```python
from build123d import *

# Parameters (mm, degrees)
F0_R     = 10.5
F1_DEPTH = 1
F2_DEPTH = 50
F3_R     = 5
F5_DEPTH = 51
F6_R     = 0.5


with BuildPart() as f1:
    # F0 (on Top) → F1 (new body)
    with BuildSketch(Plane.XY):
        with BuildLine():
            ThreePointArc((11, -3.3541019662), (10.6256868339, -1.6955824958), (10.5, 0))
            ThreePointArc((10.5, 0), (10.6256868339, 1.6955824958), (11, 3.3541019662))
            ThreePointArc((11, 3.3541019662), (-11.5, 0), (11, -3.3541019662))
        make_face()
        Circle(F0_R, mode=Mode.SUBTRACT)
        with BuildLine():
            ThreePointArc((55.5, 0), (45.6955824958, 11.3743131661), (33, 3.3541019662))
            ThreePointArc((33, 3.3541019662), (33.3743131661, 1.6955824958), (33.5, 0))
            ThreePointArc((33.5, 0), (33.3743131661, -1.6955824958), (33, -3.3541019662))
            ThreePointArc((33, -3.3541019662), (45.6955824958, -11.3743131661), (55.5, 0))
        make_face()
        with BuildLine():
            ThreePointArc((54.5, 0), (44, -10.5), (33.5, 0))
            ThreePointArc((33.5, 0), (44, 10.5), (54.5, 0))
        make_face(mode=Mode.SUBTRACT)
        Circle(F0_R)
        with BuildLine():
            ThreePointArc((32.5, 0), (22, 10.5), (11.5, 0))
            ThreePointArc((11.5, 0), (22, -10.5), (32.5, 0))
        make_face()
        with BuildLine():
            ThreePointArc((54.5, 0), (44, 10.5), (33.5, 0))
            ThreePointArc((33.5, 0), (44, -10.5), (54.5, 0))
        make_face()
        with BuildLine():
            ThreePointArc((33, 3.3541019662), (22, 11.5), (11, 3.3541019662))
            ThreePointArc((11, 3.3541019662), (11.3743131661, 1.6955824958), (11.5, 0))
            ThreePointArc((11.5, 0), (22, 10.5), (32.5, 0))
            ThreePointArc((32.5, 0), (32.6256868339, 1.6955824958), (33, 3.3541019662))
        make_face()
        with BuildLine():
            ThreePointArc((11.5, 0), (11.3743131661, -1.6955824958), (11, -3.3541019662))
            ThreePointArc((11, -3.3541019662), (22, -11.5), (33, -3.3541019662))
            ThreePointArc((33, -3.3541019662), (32.6256868339, -1.6955824958), (32.5, 0))
            ThreePointArc((32.5, 0), (22, -10.5), (11.5, 0))
        make_face()
        with BuildLine():
            ThreePointArc((11, 3.3541019662), (10.6256868339, 1.6955824958), (10.5, 0))
            ThreePointArc((10.5, 0), (10.6256868339, -1.6955824958), (11, -3.3541019662))
            ThreePointArc((11, -3.3541019662), (11.3743131661, -1.6955824958), (11.5, 0))
            ThreePointArc((11.5, 0), (11.3743131661, 1.6955824958), (11, 3.3541019662))
        make_face()
        with BuildLine():
            ThreePointArc((33.5, 0), (33.3743131661, 1.6955824958), (33, 3.3541019662))
            ThreePointArc((33, 3.3541019662), (32.6256868339, 1.6955824958), (32.5, 0))
            ThreePointArc((32.5, 0), (32.6256868339, -1.6955824958), (33, -3.3541019662))
            ThreePointArc((33, -3.3541019662), (33.3743131661, -1.6955824958), (33.5, 0))
        make_face()
    extrude(amount=-F1_DEPTH)

    # F0 (on Top) → F2 (join)
    with BuildSketch(Plane.XY):
        with BuildLine():
            ThreePointArc((11, -3.3541019662), (10.6256868339, -1.6955824958), (10.5, 0))
            ThreePointArc((10.5, 0), (10.6256868339, 1.6955824958), (11, 3.3541019662))
            ThreePointArc((11, 3.3541019662), (-11.5, 0), (11, -3.3541019662))
        make_face()
        Circle(F0_R, mode=Mode.SUBTRACT)
        with BuildLine():
            ThreePointArc((11, 3.3541019662), (10.6256868339, 1.6955824958), (10.5, 0))
            ThreePointArc((10.5, 0), (10.6256868339, -1.6955824958), (11, -3.3541019662))
            ThreePointArc((11, -3.3541019662), (11.3743131661, -1.6955824958), (11.5, 0))
            ThreePointArc((11.5, 0), (11.3743131661, 1.6955824958), (11, 3.3541019662))
        make_face()
        with BuildLine():
            ThreePointArc((33, 3.3541019662), (22, 11.5), (11, 3.3541019662))
            ThreePointArc((11, 3.3541019662), (11.3743131661, 1.6955824958), (11.5, 0))
            ThreePointArc((11.5, 0), (22, 10.5), (32.5, 0))
            ThreePointArc((32.5, 0), (32.6256868339, 1.6955824958), (33, 3.3541019662))
        make_face()
        with BuildLine():
            ThreePointArc((11.5, 0), (11.3743131661, -1.6955824958), (11, -3.3541019662))
            ThreePointArc((11, -3.3541019662), (22, -11.5), (33, -3.3541019662))
            ThreePointArc((33, -3.3541019662), (32.6256868339, -1.6955824958), (32.5, 0))
            ThreePointArc((32.5, 0), (22, -10.5), (11.5, 0))
        make_face()
        with BuildLine():
            ThreePointArc((33.5, 0), (33.3743131661, 1.6955824958), (33, 3.3541019662))
            ThreePointArc((33, 3.3541019662), (32.6256868339, 1.6955824958), (32.5, 0))
            ThreePointArc((32.5, 0), (32.6256868339, -1.6955824958), (33, -3.3541019662))
            ThreePointArc((33, -3.3541019662), (33.3743131661, -1.6955824958), (33.5, 0))
        make_face()
        with BuildLine():
            ThreePointArc((55.5, 0), (45.6955824958, 11.3743131661), (33, 3.3541019662))
            ThreePointArc((33, 3.3541019662), (33.3743131661, 1.6955824958), (33.5, 0))
            ThreePointArc((33.5, 0), (33.3743131661, -1.6955824958), (33, -3.3541019662))
            ThreePointArc((33, -3.3541019662), (45.6955824958, -11.3743131661), (55.5, 0))
        make_face()
        with BuildLine():
            ThreePointArc((54.5, 0), (44, -10.5), (33.5, 0))
            ThreePointArc((33.5, 0), (44, 10.5), (54.5, 0))
        make_face(mode=Mode.SUBTRACT)
    extrude(amount=F2_DEPTH)

    # F3
    f3_edges = [f1.edges().sort_by_distance(p)[0] for p in [
        (11, 3.354102, 24.5),
        (33, 3.354102, 24.5),
        (11, -3.354102, 24.5),
        (33, -3.354102, 24.5),
    ]]
    fillet(f3_edges, radius=F3_R)

    # F4 (on face) → F5 (cut, through all)
    with BuildSketch(Plane.XY.offset(50)):
        with BuildLine():
            Line((-8.6168439698, -6), (-9.8107084352, -6))
            ThreePointArc((-9.8107084352, -6), (-1.674067678, -11.3774996115), (7.6666666667, -8.5715939137))
            add(Edge.make_bspline(
                [(7.6666666667, -8.5715939137), (7.8739148264, -8.3862255244), (8.0987281428, -8.2100412723), (8.3407825678, -8.0456674851), (8.5991550728, -7.8958830707), (8.8721389341, -7.7633595184), (9.4430101632, -7.5370516436), (9.7409333736, -7.4433205753), (10.0487851549, -7.3712866338), (10.3635540468, -7.3226772778), (10.6817776263, -7.2983738762), (11.3169501229, -7.2983738762), (11.6339014321, -7.3224833437), (11.9474393092, -7.3707047572), (12.2541428107, -7.4421708702), (12.5510327606, -7.5351814239), (13.1223942737, -7.760709488), (13.3967057595, -7.8934858401), (13.6563094067, -8.0436938162), (13.8994714876, -8.2086307147), (14.1252554599, -8.3854834059), (14.3333333333, -8.5715939137)],
                knots=[0, 0, 0, 0, 0, 0, 0, 0.2498284224, 0.2498284224, 0.2498284224, 0.2498284224, 0.2498284224, 0.4999999993, 0.4999999993, 0.4999999993, 0.4999999993, 0.4999999993, 0.749171392, 0.749171392, 0.749171392, 0.749171392, 0.749171392, 1, 1, 1, 1, 1, 1, 1], degree=6))
            ThreePointArc((14.3333333333, -8.5715939137), (22, -11.5), (29.6666666667, -8.5715939137))
            add(Edge.make_bspline(
                [(36.3333333333, -8.5715939137), (36.1260851736, -8.3862255244), (35.9012718572, -8.2100412723), (35.6592174322, -8.0456674851), (35.4008449272, -7.8958830707), (35.1278610659, -7.7633595184), (34.5569898368, -7.5370516436), (34.2590666264, -7.4433205753), (33.9512148451, -7.3712866338), (33.6364459532, -7.3226772778), (33.3182223737, -7.2983738762), (32.6830498771, -7.2983738762), (32.3660985679, -7.3224833437), (32.0525606908, -7.3707047572), (31.7458571893, -7.4421708702), (31.4489672394, -7.5351814239), (30.8776057263, -7.760709488), (30.6032942405, -7.8934858401), (30.3436905933, -8.0436938162), (30.1005285124, -8.2086307147), (29.8747445401, -8.3854834059), (29.6666666667, -8.5715939137)],
                knots=[0, 0, 0, 0, 0, 0, 0, 0.2498284224, 0.2498284224, 0.2498284224, 0.2498284224, 0.2498284224, 0.4999999993, 0.4999999993, 0.4999999993, 0.4999999993, 0.4999999993, 0.749171392, 0.749171392, 0.749171392, 0.749171392, 0.749171392, 1, 1, 1, 1, 1, 1, 1], degree=6))
            ThreePointArc((36.3333333333, -8.5715939137), (45.674067678, -11.3774996115), (53.8107084352, -6))
            Line((53.8107084352, -6), (52.6168439698, -6))
            ThreePointArc((52.6168439698, -6), (44, -10.5), (35.3831560302, -6))
            Line((35.3831560302, -6), (30.6168439698, -6))
            ThreePointArc((30.6168439698, -6), (22, -10.5), (13.3831560302, -6))
            Line((13.3831560302, -6), (8.6168439698, -6))
            ThreePointArc((8.6168439698, -6), (0, -10.5), (-8.6168439698, -6))
        make_face()
        with BuildLine():
            Line((8.6168439698, -6), (-8.6168439698, -6))
            ThreePointArc((-8.6168439698, -6), (0, -10.5), (8.6168439698, -6))
        make_face()
        with BuildLine():
            Line((30.6168439698, -6), (13.3831560302, -6))
            ThreePointArc((13.3831560302, -6), (22, -10.5), (30.6168439698, -6))
        make_face()
        with BuildLine():
            ThreePointArc((35.3831560302, -6), (44, -10.5), (52.6168439698, -6))
            Line((52.6168439698, -6), (35.3831560302, -6))
        make_face()
    extrude(amount=-F5_DEPTH, mode=Mode.SUBTRACT)

    # F6
    f6_edges = [f1.edges().sort_by_distance(p)[0] for p in [
        (-8.616844, -6, 25),
        (8.616844, -6, 25),
        (13.383156, -6, 25),
        (30.616844, -6, 25),
        (35.383156, -6, 25),
        (52.616844, -6, 25),
    ]]
    fillet(f6_edges, radius=F6_R)


solid = f1.part
```
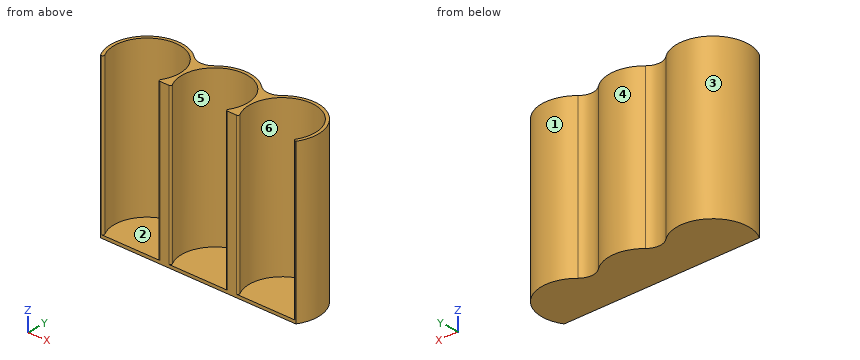
Source: CAD feature listing. Evaluate the final solid. Frame: model axes, mm. Face numbers are marked on the shaded views. A direction names the side the tool comes from. Round coordinates to 2 decimals unless told otherwise and drop trailing zeros. Write each loop counter-clockwise with the first axis right and the second up, starting at its lowest first coordinate (ties: lowest second). Pieces come first, ordered by that corner, then holes. Notation, with made-up numbers: M 28.25,50 L 87.25,50 A18 ccw 87.25,82 Z; hole C 39,-3 d1. An arc over 180 degrees is marked long. Answer as a JSON object with one key per item and string values. Group by question number.
(1) First-contact query: pin 1 (1.5 mm diameter, centred on x = 47, y = -1.5, fed in from +Z); pin 2 (1 mm diameter, centred on y = 7.5, z = 14.5, fed in from -X); pin 3 (5 mm diameter, centred on y = 9.5, z = 20, fed in from +X). Flat tips, straight axial feed; report the tip coordinate or a pass-through.
(2) Reachability of the marked faces 1 and 2 from +Z, -Z, +X, -X, +Y, -Y: full face, straight path, thin tool, end or side. Return the list, or none.
(3) Section query B-B on x = 44. Output: boundary loops of the cut face in (y, z).
(4) Section query C-C on x = 27.5. Output: boundary loops of the cut face in (y, z).
(5) Ray query, line 1 (X direction, y = 0, z = 15.5); line 2 (Z direction, x = 45.5, y = 10.25); line 3 (X direction, y = -1.5, z = 20.5). Return the intervals inside material, ascending. Write a range as [from, to].
(6) Mould query, pull axis Y, two halves, no side actions, for the marked faces 3, 4, 5 and 6. Classes: +Y half, -Y half, draft (parallel to the pull), parting line (faces both ways), or undercut.
(7) Section query A-A on y = -1.75. Output: boundary loops of the cut face in (x, z).
Computed values:
{
 "1": {"pin 1": "z = 0", "pin 2": "x = -9.12", "pin 3": "x = 53.12"},
 "2": {"face 1": "+Z, -Z", "face 2": "+Z"},
 "3": {"outline": "M -6,-1 L 11.5,-1 L 11.5,50 L 10.5,50 L 10.5,0 L -6,0 Z"},
 "4": {"outline": "M -6,-1 L 10.1,-1 L 10.1,50 L 8.94,50 L 8.94,0 L -6,0 Z"},
 "5": {"line 1": "[-11.5, -10.5], [10.5, 11.5], [32.5, 33.5], [54.5, 55.5]", "line 2": "[-1, 0]", "line 3": "[-11.4, -10.39], [10.39, 11.61], [32.39, 33.61], [54.39, 55.4]"},
 "6": {"face 3": "parting line", "face 4": "+Y half", "face 5": "undercut", "face 6": "undercut"},
 "7": {"outline": "M -11.37,-1 L 55.37,-1 L 55.37,50 L 54.35,50 L 54.35,0 L 33.65,0 L 33.65,50 L 32.35,50 L 32.35,0 L 11.65,0 L 11.65,50 L 10.35,50 L 10.35,0 L -10.35,0 L -10.35,50 L -11.37,50 Z"}
}
